Read the model definition and answer for the solid it produces. Units are mm, in the model's axes. Coordinates: 2 decimals unless noted, no trailing zeros. Order: outer loops, then holes, each group sorted by start corner. A loop starts at its lowest first (then second) coordinate and runs counter-clockwise, first axis right, second up. Notation, with made-up numbers: (76, -11.5) -> (133, -11.5) arc R36 ccw to (133, 27.5) -> close; hole circle Ø4 at (73, -6.75). An arc over 180 degrees is marked (long way). Answer as a JSON object with one key per item and string values. Group by question number.
1) Section C-C on y = 39 is taken. Determine the outline of the cut face in (x, z).
2) Consider L1, parallel to Y at x = 19.5, z = 1.3; L2, parallel to X at y = 32, z = 1.3; L3, parallel to Y at x = 142, z = 2.7. Determine where each line is inside the solid, lowest interval first.
3) Section A-A on z = 2.1 is taken. Determine the outline of the cut face in (x, y).
4) Given pin 1 (1.5 mm diameter, centred on x = 184.5, z = 1, fed in from -Y); pin 2 (1.5 mm diameter, centred on x = 263.5, z = 0.5, fed in from -Y); pin 3 (1.5 mm diameter, centred on y = 46.5, z = 2, fed in from +X), each flat-ended and moving along its own axis, determine where each tip first touches the part or whether it passes through.
5) Section B-B on x = 174 is taken. Determine the outline of the cut face in (y, z).
Autodesk Inventor part; units mm, degrees
ref_plane "YZ Plane" through (0, 0, 0) normal (1, 0, 0) x (0, 1, 0)
ref_plane "XZ Plane" through (0, 0, 0) normal (0, 1, 0) x (-1, 0, 0)
ref_plane "XY Plane" through (0, 0, 0) normal (0, 0, 1) x (1, 0, 0)
sketch "Skizze1" plane through (0, 0, 0) normal (0, 0, 1) x (1, 0, 0)
  line L0 (-71, 0) -> (391, 0)
  line L1 (-5, 35) -> (-5, 30)
  line L2 (-5, 30) -> (229.7825, 10)
  line L3 (325, 70) -> (325, 110)
  line L4 (325, 110) -> (-5, 35)
  arc A0 (325, 70) -> (229.7825, 10) centre (325, -35.5531) ccw
  line L5 (325, 90) -> (237, 90)
  point P0 (0, 0)
  dimension "d3" = 5
  dimension "d5" = 330
  dimension "d6" = 40
  dimension "d7" = 5
  dimension "d8" = 30
  dimension "d9" = 230
  dimension "d13" = 10
  dimension "d14" = 70
extrude "Extrusion1" add sketch "Skizze1" along normal blind 3 contours L4 L5 L3 A0 L2 L1
equation "\"G_L\" = 0"
equation "\"G_H\" = 0"
equation "\"G_B\" = 0"
properties part number "Center_fin" material "GEDA Polyamid"
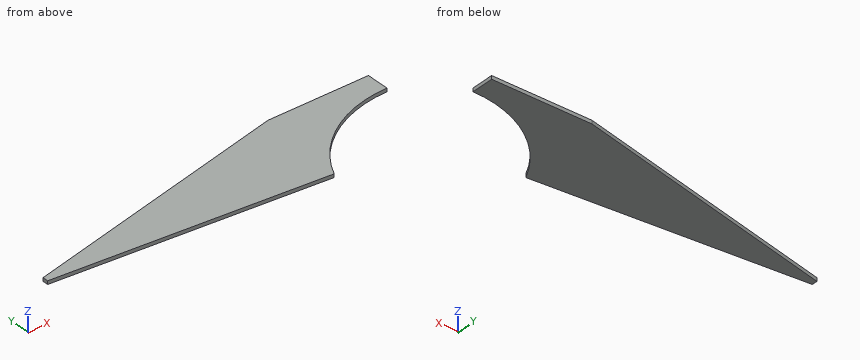
Worked answers:
{
 "1": {"outline": "(12.6, 0) -> (250.28, 0) -> (250.28, 3) -> (12.6, 3) -> close"},
 "2": {"L1": "y = 27.91 to 40.57", "L2": "x = -5 to 243.89", "L3": "y = 17.48 to 68.41"},
 "3": {"outline": "(-5, 30) -> (229.78, 10) arc R105.55 cw to (325, 70) -> (325, 90) -> (237, 90) -> (-5, 35) -> close"},
 "4": {"pin 1": "stops at y = 13.79", "pin 2": "stops at y = 49.69", "pin 3": "stops at x = 259.54"},
 "5": {"outline": "(14.75, 0) -> (75.68, 0) -> (75.68, 3) -> (14.75, 3) -> close"}
}
